Read the model definition and answer for the solid it produces. Units are mm, in the model's axes. Face numbers are marked on the shaded views. A direction names the side the tool comes from. Round coordinates to 2 decimals unless told otherwise and drop trailing zeros. Write each loop counter-clockwise with the first axis right and the second up, starting at its lowest first coordinate (ties: lowest second). Pieces come first, ordered by that corner, then holes. Notation, with made-up numbers: (-15, 70.25) - (37, 70.25) arc R9 ccw to (37, 84.25) - close; hole circle Ø3 at (65.25, 18). An arc over 180 degrees is marked (long way). Use one line per item in the form item = value. Start each with the question number.
1) Each of these flat-tipped pins is pushed along its axis until it touches: pin 1 (0.6 mm diameter, centred on x = 18.5, z = 9.5, fed in from +Y); pin 2 (0.6 mm diameter, centred on x = 13.5, z = 9, fed in from -Y); pin 3 (0.6 mm diameter, centred on y = 1.5, z = 7.5, fed in from +X). Where does it stop, or does it pass through?
2) The part is cut by section D-D, the plane x = 18. Give the vertices of the cut face in (y, z), plus the area to 4 significant figures.
3) The part is cut by section C-C, the plane y = 14. Give the vertices of the cut face in (x, z).
4) Consider line 1 along X through (y, z) = (14, 1.4); line 2 along Y through (x, z) = (2, 1.45); line 3 along Z through (x, y) = (17.25, 2.75). Determine where each line is inside the solid, lowest interval first. Write a range as from..to.
5) The part is cut by section B-B, the plane z = 4.75. Count the separate pieces of the cut face and the enclosed holes in it, plus the area to 3 significant figures.
6) For a pull along X with two mould halves and no side action, classify the marked faces 1, 2, 3 and 4 as released by +X, released by -X, zero draft, split by the parting line, or undercut.
7) The part is cut by section A-A, the plane x = 2.75. Give the vertices of the cut face in (y, z), plus the area to 4 significant figures.
8) For the marked faces 5 and 6, determine the directions among +Z, -Z, +X, -X, +Y, -Y from which every point of the face is accessible in a straight line to the end or side of a thin tool.
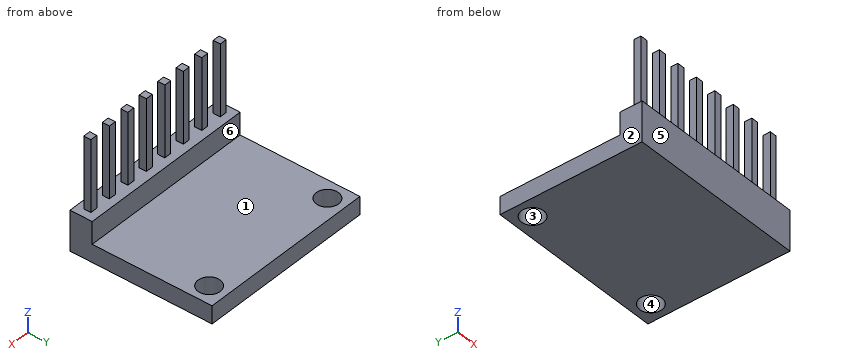
Autodesk Inventor part; units mm, degrees
ref_plane "YZ Plane" through (0, 0, 0) normal (1, 0, 0) x (0, 1, 0)
ref_plane "XZ Plane" through (0, 0, 0) normal (0, 1, 0) x (-1, 0, 0)
ref_plane "XY Plane" through (0, 0, 0) normal (0, 0, 1) x (1, 0, 0)
sketch "Esquisse1" plane through (0, 0, 0) normal (0, 0, 1) x (1, 0, 0)
  line L0 (0, 16) -> (20, 16)
  line L1 (20, 16) -> (20, 0)
  line L2 (20, 0) -> (0, 0)
  line L3 (0, 0) -> (0, 16)
  line L4 (-4.5575, 0) -> (27.3449, 0)
  line L5 (0, -3.2) -> (0, 19.2)
  point P0 (0, 0)
  dimension "d0" = 20
  dimension "d1" = 16
extrude "Extrusion1" add sketch "Esquisse1" along normal blind 2
sketch "Esquisse2" plane through (0, 0, 2) normal (0, 0, 1) x (1, 0, 0)
  line L0 (20, 0) -> (20, 16)
  line L1 (20, 16) -> (0, 16)
  line L2 (0, 16) -> (0, 0)
  point P0 (2, 14)
  point P1 (18, 14)
  dimension "d11" = 2
  dimension "d12" = 2
  dimension "d13" = 2
  dimension "d14" = 2
hole "Perçage1" at (2, 14, 2) at (18, 14, 2) direction (0, 0, -1) diameter 2.5 end through all
sketch "Esquisse3" plane through (0, 0, 2) normal (0, 0, 1) x (1, 0, 0)
  line L0 (0, 2.5) -> (2.5, 2.5)
  line L1 (2.5, 2.5) -> (2.5, 0)
  line L2 (2.5, 0) -> (0, 0)
  line L3 (0, 0) -> (0, 2.5)
  line L4 (-4.5575, 0) -> (27.3449, 0)
  line L5 (2.5, 2.5) -> (5, 2.5)
  line L6 (5, 2.5) -> (5, 0)
  line L7 (5, 0) -> (2.5, 0)
  line L8 (2.5, 0) -> (2.5, 2.5)
  line L9 (5, 2.5) -> (7.5, 2.5)
  line L10 (7.5, 2.5) -> (7.5, 0)
  line L11 (7.5, 0) -> (5, 0)
  line L12 (5, 0) -> (5, 2.5)
  line L13 (7.5, 2.5) -> (10, 2.5)
  line L14 (10, 2.5) -> (10, 0)
  line L15 (10, 0) -> (7.5, 0)
  line L16 (7.5, 0) -> (7.5, 2.5)
  line L17 (10, 2.5) -> (12.5, 2.5)
  line L18 (12.5, 2.5) -> (12.5, 0)
  line L19 (12.5, 0) -> (10, 0)
  line L20 (10, 0) -> (10, 2.5)
  line L21 (12.5, 2.5) -> (15, 2.5)
  line L22 (15, 2.5) -> (15, 0)
  line L23 (15, 0) -> (12.5, 0)
  line L24 (12.5, 0) -> (12.5, 2.5)
  line L25 (15, 2.5) -> (17.5, 2.5)
  line L26 (17.5, 2.5) -> (17.5, 0)
  line L27 (17.5, 0) -> (15, 0)
  line L28 (15, 0) -> (15, 2.5)
  line L29 (17.5, 2.5) -> (20, 2.5)
  line L30 (20, 2.5) -> (20, 0)
  line L31 (20, 0) -> (17.5, 0)
  line L32 (17.5, 0) -> (17.5, 2.5)
  line L33 (0, 16) -> (0, 0)
  line L34 (0, 0) -> (20, 0)
  point P0 (2.5, 0)
  point P1 (20, 0)
  dimension "d15" = 2.5
  dimension "d16" = 2.5
  dimension "d19" = 2.5
extrude "Extrusion2" add sketch "Esquisse3" along normal blind 2.5
sketch "Esquisse4" plane through (0, 0, 4.5) normal (0, 0, 1) x (1, 0, 0)
  line L0 (0.8, 1.6) -> (1.6, 1.6)
  line L1 (1.6, 1.6) -> (1.6, 0.8)
  line L2 (1.6, 0.8) -> (0.8, 0.8)
  line L3 (0.8, 0.8) -> (0.8, 1.6)
  line L4 (0, 0) -> (20, 0)
  line L5 (0, 2.5) -> (0, 0)
  line L6 (3.3, 1.6) -> (4.1, 1.6)
  line L7 (4.1, 1.6) -> (4.1, 0.8)
  line L8 (4.1, 0.8) -> (3.3, 0.8)
  line L9 (3.3, 0.8) -> (3.3, 1.6)
  line L10 (5.8, 1.6) -> (6.6, 1.6)
  line L11 (6.6, 1.6) -> (6.6, 0.8)
  line L12 (6.6, 0.8) -> (5.8, 0.8)
  line L13 (5.8, 0.8) -> (5.8, 1.6)
  line L14 (8.3, 1.6) -> (9.1, 1.6)
  line L15 (9.1, 1.6) -> (9.1, 0.8)
  line L16 (9.1, 0.8) -> (8.3, 0.8)
  line L17 (8.3, 0.8) -> (8.3, 1.6)
  line L18 (10.8, 1.6) -> (11.6, 1.6)
  line L19 (11.6, 1.6) -> (11.6, 0.8)
  line L20 (11.6, 0.8) -> (10.8, 0.8)
  line L21 (10.8, 0.8) -> (10.8, 1.6)
  line L22 (13.3, 1.6) -> (14.1, 1.6)
  line L23 (14.1, 1.6) -> (14.1, 0.8)
  line L24 (14.1, 0.8) -> (13.3, 0.8)
  line L25 (13.3, 0.8) -> (13.3, 1.6)
  line L26 (15.8, 1.6) -> (16.6, 1.6)
  line L27 (16.6, 1.6) -> (16.6, 0.8)
  line L28 (16.6, 0.8) -> (15.8, 0.8)
  line L29 (15.8, 0.8) -> (15.8, 1.6)
  line L30 (18.3, 1.6) -> (19.1, 1.6)
  line L31 (19.1, 1.6) -> (19.1, 0.8)
  line L32 (19.1, 0.8) -> (18.3, 0.8)
  line L33 (18.3, 0.8) -> (18.3, 1.6)
  point P0 (0, 1.25)
  dimension "d26" = 0.8
  dimension "d27" = 0.8
  dimension "d28" = 0.8
  dimension "d29" = 0.8
  dimension "d32" = 2.5
extrude "Extrusion3" add sketch "Esquisse4" along normal blind 8
equation "\"d16\" = d15"
equation "\"d27\" = d26"
properties part number "gyro"
Geometry results:
q1.pin_1 = 1.6
q1.pin_2 = 0.8
q1.pin_3 = 19.1
q2.outline = (0, 0) - (12.75, 0) - (12.75, 2) - (2.5, 2) - (2.5, 4.5) - (0, 4.5) - close; (15.25, 0) - (16, 0) - (16, 2) - (15.25, 2) - close
q2.area = 33.25 mm2
q3.outline = (0, 0) - (0.75, 0) - (0.75, 2) - (0, 2) - close; (3.25, 0) - (16.75, 0) - (16.75, 2) - (3.25, 2) - close; (19.25, 0) - (20, 0) - (20, 2) - (19.25, 2) - close
q4.line_1 = 0..0.75, 3.25..16.75, 19.25..20
q4.line_2 = 0..12.75, 15.25..16
q4.line_3 = 0..2
q5.separate_pieces = 8
q5.enclosed_holes = 0
q5.area = 5.12 mm2
q6.face_1 = zero draft
q6.face_2 = released by -X
q6.face_3 = undercut
q6.face_4 = undercut
q7.outline = (0, 0) - (13, 0) - (13, 2) - (2.5, 2) - (2.5, 4.5) - (0, 4.5) - close; (15, 0) - (16, 0) - (16, 2) - (15, 2) - close
q7.area = 34.25 mm2
q8.face_5 = +Z, -Z, +X, -X, -Y
q8.face_6 = +Z, +X, -X, +Y
